The listing builds one solid part. Answer for the finished solid, in the listing's coordinates (mm). A direction names the side the tool comes from. Give positions to 0.01 mm unless a question says otherwise; leave off trailing zeros. Write each loop counter-clockwise with the first axis right and the second up, starting at its lowest first coordinate (ties: lowest second). Pieces come first, ordered by that corner, then holes. Notation, with made-up numbers: (45.5, 0.5) - (71.5, 0.5) arc R20 cw to (71.5, 13.5) - close; hole circle Ø5 at (-26.5, 21). An arc over 180 degrees is marked (long way). Write each question's results on one line, items separated by ' | '. Start each with the question number.
Q1. Section D-D (y = 17.5) is taken. Determine the outline of the cut face in (x, z), plus the area to 3 significant figures.
Q2. Section B-B (x = 0) is taken. Determine the outline of the cut face in (y, z) (3 decimals), plus the area to 3 significant figures.
Q3. For faces 1 (the face through (-18, 12.7, -22)), 2 (the face through (15.2, -1, 19)), 3 (the face through (2, 4.61, 15)), 4 (the face through (16, 12.96, 1)), determine the directions among +Z, -Z, +X, -X, +Y, -Y from which every point of the face is accessible in a straight line to the end or side of a thin tool.
Q4. Flat-ended cylindrical pins translate along their axes: pin 1 Ø4 at (y, z) = (10, -18.5) entering from +X; pin 2 Ø6.5 at (y, z) = (-3, 18.5) entering from +X; pin 3 Ø1.3 at (x, z) = (-16.5, 5) entering from +Y; pin 4 Ø11.5 at (x, z) = (0.5, 12.5) entering from +Y. Find the tip coordinate at first contact, or state that the pin passes through.
Q5. Find the intervals of material crossed by probe 1 along Z at (x, y) = (0, -3.75); probe 2 along Z at (x, y) = (0, 6.5); probe 3 along X at (y, z) = (25, 6), in increasing order.
Q6. For a pull along Y with two mould halves and no side action, classify faces 5 (the face through (-17.74, 11.33, 15.18)), 6 (the face through (20.206, 5, -4)), 7 (the face through (19, 27.305, 6)) as pulls with the +Y half, pulls with the -Y half, needs draft (parallel to the pull), parting line crosses it, or undercut.
Q7. Section C-C (y = 1.5) is taken. Determine the outline of the cut face in (x, z).
Q8. Section A-A (y = 10.16) is taken. State how many separate pieces and enclosed holes the cut face has, plus the area to 3 significant figures.
```python
from build123d import *

# Parameters (mm, degrees)
SKETCH1_W                       = 45.72
SKETCH1_H                       = 60.96
BOSS_EXTRUDE1_DEPTH             = 6.35
SKETCH2_W                       = 7.6600046
SKETCH2_H                       = 60.96
BOSS_EXTRUDE2_DEPTH             = 20.955
LPATTERN1_COUNT                 = 3
LPATTERN1_PITCH                 = 17.018
SKETCH1_3_W                     = 45.72
SKETCH1_3_H                     = 60.96
BOSS_EXTRUDE3_DEPTH             = 2.54
CUT_EXTRUDE1_START              = 15.199995
SKETCH11_W                      = 60.96
SKETCH11_H                      = 14.3449802
CUT_EXTRUDE1_DEPTH              = 17.78
CUT_EXTRUDE2_DEPTH              = 62.358877312
SKETCH17_W                      = 45.72
SKETCH17_H                      = 60.96
BOSS_EXTRUDE4_DEPTH             = 6.785
SKETCH19_W                      = 30.3999908
SKETCH19_H                      = 60.96
BOSS_EXTRUDE5_DEPTH             = 1.0100056
CBORE_FOR_M5_SBHCS2_D           = 5.5
CBORE_FOR_M5_SBHCS2_CBORE_D     = 10.5
CBORE_FOR_M5_SBHCS2_CBORE_DEPTH = 2.75
CUT_EXTRUDE3_DEPTH              = 82.222264916
CUT_EXTRUDE3_DEPTH_BACK         = 82.222264916
SKETCH24_W                      = 5.08
SKETCH24_H                      = 45.72
SKETCH25_W                      = 7.6600046
SKETCH25_H                      = 36.63
CUT_EXTRUDE4_DEPTH              = 12.7
SKETCH26_W                      = 2.400000026
SKETCH26_H                      = 36.63
CUT_EXTRUDE5_DEPTH              = 67.262485805
SKETCH27_W                      = 2.5
SKETCH27_H                      = 36.63
CUT_EXTRUDE6_DEPTH              = 67.262485805
CHAMFER1_SIZE                   = 2.5
SKETCH28_W                      = 0.254
SKETCH28_H                      = 36.63
CUT_EXTRUDE7_DEPTH              = 66.473269538


with BuildPart() as part:
    # Sketch1 → Boss-Extrude1 (new body)
    with BuildSketch(Plane(origin=(0, 0, 0), x_dir=(1, 0, 0), z_dir=(0, 1, 0))):
        Rectangle(SKETCH1_W, SKETCH1_H)
    extrude(amount=BOSS_EXTRUDE1_DEPTH)

    # Sketch2 → Boss-Extrude2 (add)
    with BuildSketch(Plane(origin=(0, 6.35, 0), x_dir=(1, 0, 0), z_dir=(0, 1, 0))):
        with Locations((-19.0299977, 0)):
            Rectangle(SKETCH2_W, SKETCH2_H)
        with Locations((19.0299977, 0)):
            Rectangle(SKETCH2_W, SKETCH2_H)
    extrude(amount=BOSS_EXTRUDE2_DEPTH)

    # Sketch7 → M2 Clearance Hole2 (revolve, cut)
    with BuildSketch(Plane(origin=(22.86, 10.16, 14.9171914), x_dir=(0, 0, -1), z_dir=(0, 1, 0))):
        Polygon((0, 0), (0, 46.441032743), (1.2, 45.72), (1.2, 0), align=None)
    m2_clearance_hole2 = revolve(axis=Axis((29.21, 10.16, 14.9171914), (-1, 0, 0)), mode=Mode.SUBTRACT)

    # LPattern1: M2 Clearance Hole2 ×3
    with Locations(*[(0, 0, -i * LPATTERN1_PITCH) for i in range(1, LPATTERN1_COUNT)]):
        add(m2_clearance_hole2, mode=Mode.SUBTRACT)

    # Sketch1<3> → Boss-Extrude3 (add)
    with BuildSketch(Plane(origin=(0, 0, 0), x_dir=(1, 0, 0), z_dir=(0, 1, 0))):
        Rectangle(SKETCH1_3_W, SKETCH1_3_H)
    extrude(amount=-BOSS_EXTRUDE3_DEPTH)

    # Sketch11 → Cut-Extrude1 (cut, symmetric)
    with BuildSketch(Plane.ZY.offset(-15.1999954).offset(CUT_EXTRUDE1_START)):
        with Locations((0, 20.1325099)):
            Rectangle(SKETCH11_W, SKETCH11_H)
    extrude(amount=CUT_EXTRUDE1_DEPTH, both=True, mode=Mode.SUBTRACT)

    # Sketch12 → Cut-Extrude2 (cut, through all)
    with BuildSketch(Plane(origin=(22.86, 0, 0), x_dir=(0, 0, -1), z_dir=(1, 0, 0))):
        with BuildLine():
            Line((13.105000048, 12.7), (30.48, 12.7))
            Line((30.48, 12.7), (30.48, 27.305))
            Line((30.48, 27.305), (25.661312206, 27.305))
            ThreePointArc((25.661312206, 27.305), (3.474748234, 33.679387055), (13.105000048, 12.7))
        make_face()
    extrude(amount=-CUT_EXTRUDE2_DEPTH, mode=Mode.SUBTRACT)

    # Sketch17 → Boss-Extrude4 (add)
    with BuildSketch(Plane.XZ.offset(2.54)):
        Rectangle(SKETCH17_W, SKETCH17_H)
    extrude(amount=BOSS_EXTRUDE4_DEPTH)

    # Sketch19 → Boss-Extrude5 (add)
    with BuildSketch(Plane(origin=(0, 6.35, 0), x_dir=(1, 0, 0), z_dir=(0, 1, 0))):
        Rectangle(SKETCH19_W, SKETCH19_H)
    extrude(amount=BOSS_EXTRUDE5_DEPTH)

    # CBORE for M5 SBHCS2 (through all)
    with Locations(Plane(origin=(0, 7.3600056, 0), x_dir=(1, 0, 0), z_dir=(0, 1, 0))):
        with Locations((0, -12.7), (0, 19.05)):
            CounterBoreHole(CBORE_FOR_M5_SBHCS2_D / 2, CBORE_FOR_M5_SBHCS2_CBORE_D / 2, CBORE_FOR_M5_SBHCS2_CBORE_DEPTH)

    # Sketch24 → Cut-Extrude3 (cut, two sides: drawn at the far end of the back side and taken through both)
    with BuildSketch(Plane(origin=(31.571183672, -12.7, -14.6188086), x_dir=(0, 0, -1), z_dir=(0, 1, 0)).offset(-CUT_EXTRUDE3_DEPTH_BACK)):
        with Locations((-42.5588086, 31.571183672)):
            Rectangle(SKETCH24_W, SKETCH24_H)
    extrude(amount=CUT_EXTRUDE3_DEPTH + CUT_EXTRUDE3_DEPTH_BACK, mode=Mode.SUBTRACT)

    # Sketch25 → Cut-Extrude4 (cut)
    with BuildSketch(Plane.XY.offset(25.4)):
        with Locations((19.0299977, 8.99)):
            Rectangle(SKETCH25_W, SKETCH25_H)
    extrude(amount=-CUT_EXTRUDE4_DEPTH, mode=Mode.SUBTRACT)

    # Sketch26 → Cut-Extrude5 (cut, through all)
    with BuildSketch(Plane.XY.offset(25.4)):
        with Locations((21.659999987, 8.99)):
            Rectangle(SKETCH26_W, SKETCH26_H)
    extrude(amount=-CUT_EXTRUDE5_DEPTH, mode=Mode.SUBTRACT)

    # Sketch27 → Cut-Extrude6 (cut, through all)
    with BuildSketch(Plane.XY.offset(25.4)):
        with Locations((-21.61, 8.99)):
            Rectangle(SKETCH27_W, SKETCH27_H)
    extrude(amount=-CUT_EXTRUDE6_DEPTH, mode=Mode.SUBTRACT)

    # Chamfer1
    chamfer1_edges = [part.edges().sort_by_distance(p)[0] for p in [
        (-20.36, 1.6875, -30.48),
        (-20.36, 8.99, 25.4),
    ]]
    chamfer(chamfer1_edges, length=CHAMFER1_SIZE)

    # Sketch28 → Cut-Extrude7 (cut, through all)
    with BuildSketch(Plane(origin=(0, 0, -30.48), x_dir=(-1, 0, 0), z_dir=(0, 0, -1))):
        with Locations((-20.332999974, 8.99)):
            Rectangle(SKETCH28_W, SKETCH28_H)
    extrude(amount=-CUT_EXTRUDE7_DEPTH, mode=Mode.SUBTRACT)


solid = part.part
```
Answers below:
1) outline: (-20.36, -3.16) - (-17.78, -3.16) - (-17.78, 25.4) - (-17.86, 25.4) - (-20.36, 22.9) - close; (17.78, -3.16) - (20.21, -3.16) - (20.21, 12.7) - (17.78, 12.7) - close | area: 109 mm2
2) outline: (-9.325, -30.48) - (7.36, -30.48) - (7.36, -24.3) - (4.61, -24.3) - (4.61, -21.8) - (-9.325, -21.8) - close; (-9.325, -16.3) - (4.61, -16.3) - (4.61, -13.8) - (7.36, -13.8) - (7.36, 7.45) - (4.61, 7.45) - (4.61, 9.95) - (-9.325, 9.95) - close; (-9.325, 15.45) - (4.61, 15.45) - (4.61, 17.95) - (7.36, 17.95) - (7.36, 25.4) - (-9.325, 25.4) - close | area: 721 mm2
3) face 1: -Z, +X, -X, +Y | face 2: +Z, +X, +Y, -Y | face 3: +Y | face 4: +Z, -Z, +Y
4) pin 1: stops at x = 20.21 | pin 2: stops at x = 15.2 | pin 3: stops at y = 12.96 | pin 4: stops at y = 7.36
5) probe 1: z = -30.48 to -21.8, -16.3 to 9.95, 15.45 to 25.4 | probe 2: z = -30.48 to -24.3, -13.8 to 7.45, 17.95 to 25.4 | probe 3: x = -20.36 to -17.78, 17.78 to 20.21
6) face 5: undercut | face 6: needs draft | face 7: pulls with the +Y half
7) outline: (-20.36, -27.98) - (-17.86, -30.48) - (20.21, -30.48) - (20.21, 12.7) - (15.2, 12.7) - (15.2, 25.4) - (-17.86, 25.4) - (-20.36, 22.9) - close; hole circle Ø5.5 at (0, -19.05); hole circle Ø5.5 at (0, 12.7)
8) separate pieces: 7 | enclosed holes: 0 | area: 437 mm2
